Drawing for the job (mm, zero at the part's lowest x, y, z). A direction names the side the tool comes from. Give positions to 0.01 mm unless a question says otherwise; leave off trailing zeros. Order: outer loops, then holes, each group sorted by start corner. A loop starts at its lowest first (then second) coordinate and runs counter-clockwise, first axis right, second up. Notation, with made-up numbers: (65, -34.5) - (86, -34.5) arc R13 ccw to (86, -9.5) - close; hole circle Ø11 at (4, 88). An arc over 180 degrees is marked (long way). Use a Markdown table: item, result. Add a question column.
(1) Flat gauge pins, fed straight in: pin 1 (4 mm diameter, centred on x = 2, z = 42, fed in from -Y); pin 2 (3 mm diameter, centred on y = 9.5, z = 54.5, fed in from -X). Where does each tip first touch, or does it go through?
(2) Which spindle directions (+Z, -Z, +X, -X, +Y, -Y) get a long thin tool onto all of the face, cutting with end or side? Do the marked faces 1 and 2. Say none if no direction does.
(3) Slice it at A-A (x = 6.25). Write the cut outline in (y, z).
(4) Wall check: line 1 (X direction, y = 6, z = 34.5); line 2 (Y direction, x = 6.5, z = 50.5); line 3 (X direction, y = 11, z = 44). Give the ranges that are in metal, low to high.
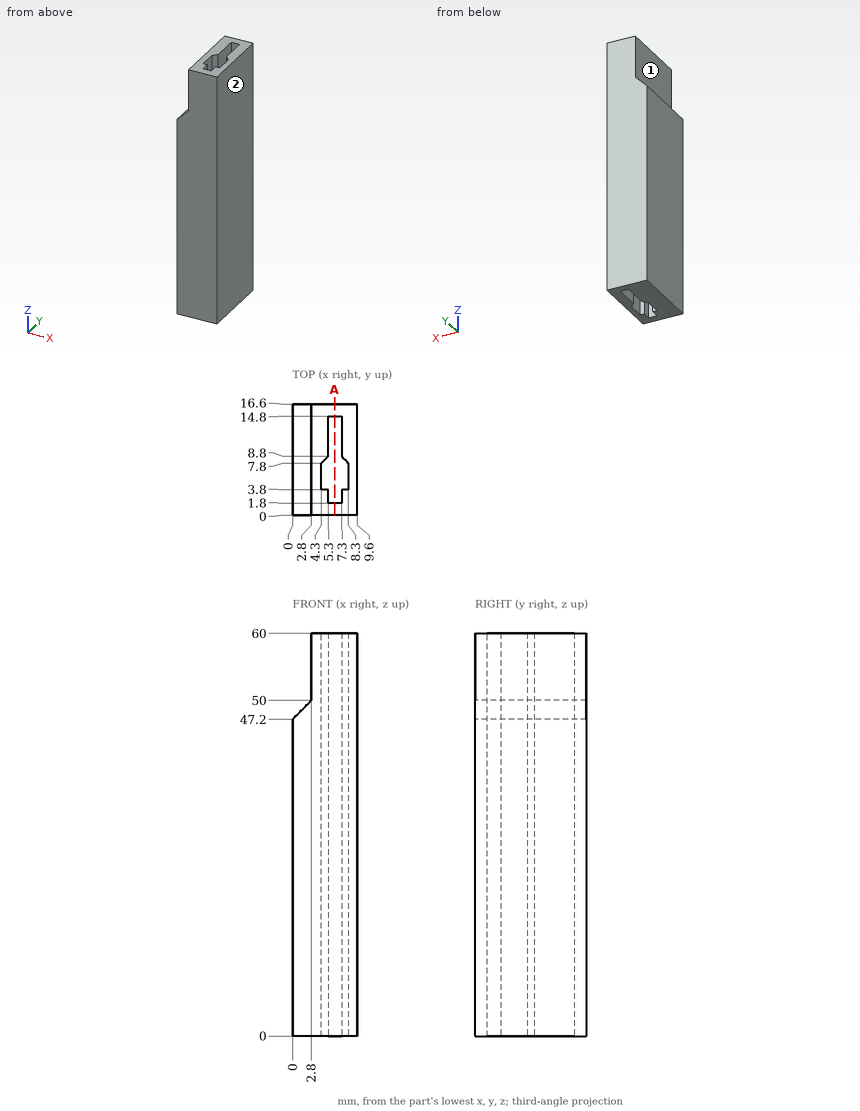
Solution:
| question | item | result |
|---|---|---|
| 1 | pin 1 | y = 0 |
| 1 | pin 2 | x = 2.8 |
| 2 | face 1 | +Z, -X, +Y, -Y |
| 2 | face 2 | +Z, -Z, +X, +Y, -Y |
| 3 | outline | (0, 0) - (1.8, 0) - (1.8, 60) - (0, 60) - close; (14.8, 0) - (16.6, 0) - (16.6, 60) - (14.8, 60) - close |
| 4 | line 1 | 0 to 4.3, 8.3 to 9.6 |
| 4 | line 2 | 0 to 1.8, 14.8 to 16.6 |
| 4 | line 3 | 0 to 5.3, 7.3 to 9.6 |
